```python
from build123d import *

# Parameters (mm, degrees)
SKETCH1_R           = 25.608746635
BOSS_EXTRUDE3_DEPTH = 4
SKETCH10_R          = 0.7
CUT_EXTRUDE1_DEPTH  = 4
SKETCH11_R          = 0.7
CUT_EXTRUDE2_DEPTH  = 4


with BuildPart() as part:
    # Sketch1 → Boss-Extrude3 (new body)
    with BuildSketch(Plane.XY):
        Circle(SKETCH1_R)
        with BuildLine():
            ThreePointArc((-18.650676838, -12), (-16.231543143, -11.700269066), (-15.931812209, -14.119402761))
            ThreePointArc((-15.931812209, -14.119402761), (-18.350945904, -14.419133695), (-18.650676838, -12))
        make_face(mode=Mode.SUBTRACT)
        with BuildLine():
            ThreePointArc((-9.804238645, -18.895954043), (-7.385104949, -18.596223108), (-7.085374015, -21.015356804))
            ThreePointArc((-7.085374015, -21.015356804), (-9.504507711, -21.315087738), (-9.804238645, -18.895954043))
        make_face(mode=Mode.SUBTRACT)
        with BuildLine():
            ThreePointArc((-22.863940025, -1.604709519), (-20.44480633, -1.304978585), (-20.145075396, -3.72411228))
            ThreePointArc((-20.145075396, -3.72411228), (-22.564209091, -4.023843215), (-22.863940025, -1.604709519))
        make_face(mode=Mode.SUBTRACT)
        with BuildLine():
            ThreePointArc((1.304978585, -20.44480633), (3.72411228, -20.145075396), (4.023843215, -22.564209091))
            ThreePointArc((4.023843215, -22.564209091), (1.604709519, -22.863940025), (1.304978585, -20.44480633))
        make_face(mode=Mode.SUBTRACT)
        with BuildLine():
            ThreePointArc((14.419133695, -18.350945904), (12, -18.650676838), (11.700269066, -16.231543143))
            ThreePointArc((11.700269066, -16.231543143), (14.119402761, -15.931812209), (14.419133695, -18.350945904))
        make_face(mode=Mode.SUBTRACT)
        with BuildLine():
            ThreePointArc((21.315087738, -9.504507711), (18.895954043, -9.804238645), (18.596223108, -7.385104949))
            ThreePointArc((18.596223108, -7.385104949), (21.015356804, -7.085374015), (21.315087738, -9.504507711))
        make_face(mode=Mode.SUBTRACT)
        with BuildLine():
            ThreePointArc((-21.315087738, 9.504507711), (-18.895954043, 9.804238645), (-18.596223108, 7.385104949))
            ThreePointArc((-18.596223108, 7.385104949), (-21.015356804, 7.085374015), (-21.315087738, 9.504507711))
        make_face(mode=Mode.SUBTRACT)
        with BuildLine():
            ThreePointArc((-11.700269066, 16.231543143), (-14.119402761, 15.931812209), (-14.419133695, 18.350945904))
            ThreePointArc((-14.419133695, 18.350945904), (-12, 18.650676838), (-11.700269066, 16.231543143))
        make_face(mode=Mode.SUBTRACT)
        with BuildLine():
            ThreePointArc((-1.304978585, 20.44480633), (-3.72411228, 20.145075396), (-4.023843215, 22.564209091))
            ThreePointArc((-4.023843215, 22.564209091), (-1.604709519, 22.863940025), (-1.304978585, 20.44480633))
        make_face(mode=Mode.SUBTRACT)
        with BuildLine():
            ThreePointArc((20.145075396, 3.72411228), (22.564209091, 4.023843215), (22.863940025, 1.604709519))
            ThreePointArc((22.863940025, 1.604709519), (20.44480633, 1.304978585), (20.145075396, 3.72411228))
        make_face(mode=Mode.SUBTRACT)
        with BuildLine():
            ThreePointArc((9.804238645, 18.895954043), (7.385104949, 18.596223108), (7.085374015, 21.015356804))
            ThreePointArc((7.085374015, 21.015356804), (9.504507711, 21.315087738), (9.804238645, 18.895954043))
        make_face(mode=Mode.SUBTRACT)
        with BuildLine():
            ThreePointArc((18.650676838, 12), (16.231543143, 11.700269066), (15.931812209, 14.119402761))
            ThreePointArc((15.931812209, 14.119402761), (18.350945904, 14.419133695), (18.650676838, 12))
        make_face(mode=Mode.SUBTRACT)
    extrude(amount=BOSS_EXTRUDE3_DEPTH)

    # Sketch9 → Revolve1 (revolve)
    with BuildSketch(Plane(origin=(0, 0, 0), x_dir=(0, 0, -1), z_dir=(1, 0, 0)), mode=Mode.PRIVATE) as revolve1_sk:
        Polygon((-32.13618734, 18.743688774), (-32.13618734, 7.487377548), (-27.00309367, 7.487377548), (-27.00309367, 18.743688774), (-27.40309367, 18.743688774), (-27.98899043, 17.487229118), (-28.78899043, 17.487229118), (-29.37488719, 18.743688774), (-29.77488719, 18.743688774), (-30.355537265, 17.498480669), (-31.155537265, 17.498480669), (-31.73618734, 18.743688774), align=None)
        Polygon((-27.00309367, 18.743688774), (-27.00309367, 7.487377548), (-21.87, 7.487377548), (-21.87, 18.743688774), (-22.27, 18.743688774), (-22.850650075, 17.498480669), (-23.650650075, 17.498480669), (-24.231300151, 18.743688774), (-24.631300151, 18.743688774), (-25.21719691, 17.487229118), (-26.01719691, 17.487229118), (-26.60309367, 18.743688774), align=None)
        Polygon((-32.13618734, 7.487377548), (-50.00618734, 7.487377548), (-50.00618734, 0), (-4, 0), (-4, 7.487377548), (-21.87, 7.487377548), (-27.00309367, 7.487377548), align=None)
    revolve(revolve1_sk.sketch.rotate(Axis((0, 0, 0), (0, 0, 1)), 90), axis=Axis((0, 0, 0), (0, 0, 1)))

    # Sketch10 → Cut-Extrude1 (cut)
    with BuildSketch(Plane.XY.offset(32.13618734)):
        with Locations((17.743688774, 0)):
            Circle(SKETCH10_R)
    extrude(amount=-CUT_EXTRUDE1_DEPTH, mode=Mode.SUBTRACT)

    # Sketch11 → Cut-Extrude2 (cut)
    with BuildSketch(Plane(origin=(0, 0, 21.87), x_dir=(-1, 0, 0), z_dir=(0, 0, -1))):
        with Locations((17.743688774, 0)):
            Circle(SKETCH11_R)
    extrude(amount=-CUT_EXTRUDE2_DEPTH, mode=Mode.SUBTRACT)


solid = part.part
```
Check sheet for the modelled part. Datum: model origin and axes. Units: mm. A direction names the side the tool comes from. Round coordinates to 2 decimals unless told otherwise and drop trailing zeros. Order: outer loops, then holes, each group sorted by start corner. A loop starts at its lowest first (then second) coordinate and runs counter-clockwise, first axis right, second up. Notation, with made-up numbers: (11, -3) - (44, -3) arc R11 ccw to (44, 5) - close; hole circle Ø2 at (-30, -26). An arc over 180 degrees is marked (long way). Answer as CSV lines item,"result". Start each with the question number.
1) Tool access check on faces 4 (the face through (-10.076, -15.805, 31.939)), 5 (the face through (8, 0, 21.87)), 6 (the face through (-19.01, -13.2, 1.97)). Record the directions out of +Z, -Z, +X, -X, +Y, -Y that give a thin tool (end or side, any length) a straight path to the whole face; none if there is none.
2) Section check B-B (z = 10). Record the cut outline in (x, y).
3) Draft check along Y on faces 1 (the face through (-10.076, -15.805, 27.009)), 2 (the face through (-17.044, 0.031, 23.842)), 3 (the face through (0, 0, 0)). Enter one of: +Y half, -Y half, draft (parallel to the pull), parting line (faces both ways), or undercut.
4) Depth check by flat-ended pin: pin 1 (1.1 mm diameter, centred on x = -17.74, y = 0, fed in from -Z); pin 2 (2 mm diameter, centred on x = -11.5, y = -15, fed in from +Z); pin 3 (10 mm diameter, centred on x = -15, z = 18.5, fed in from -Y); pin 4 (10 mm diameter, centred on y = -5.5, z = 26.5, fed in from -X). Enter the tip coordinate at first touch or a pass-through.
5) Section check A-A (y = 12.5). Give the number of separate pieces and of enclosed holes in the cut face, then the cut area to 3 significant figures.
6) Scan lines: probe 1 along Z at (x, y) = (13, 6); probe 2 along Z at (x, y) = (17.5, 6.5); probe 3 along Z at (x, y) = (-4, -17.5). Record each from-to range of solid material in increasing order.
Determined:
1,face 4,"+Z"
1,face 5,"none"
1,face 6,"+Z, -Z"
2,outline,"circle Ø14.97 at (0, 0)"
3,face 1,"parting line"
3,face 2,"undercut"
3,face 3,"draft"
4,pin 1,"z = 0"
4,pin 2,"z = 32.14"
4,pin 3,"y = -14.95"
4,pin 4,"x = -18.74"
5,separate pieces,"3"
5,enclosed holes,"0"
5,area,"433 mm^2"
6,probe 1,"0 to 4, 21.87 to 32.14"
6,probe 2,"0 to 4, 21.87 to 22.31, 24.2 to 24.67, 26.57 to 27.44, 29.34 to 29.81, 31.7 to 32.14"
6,probe 3,"0 to 4, 21.87 to 22.64, 23.86 to 25, 26.23 to 27.77, 29.01 to 30.14, 31.37 to 32.14"
